Read the model definition and answer for the solid it produces. Units are mm, in the model's axes. Face numbers are marked on the shaded views. A direction names the side the tool comes from. Coordinates: 2 decimals unless noted, no trailing zeros. Write each loop counter-clockwise with the first axis right and the second up, starting at its lowest first coordinate (ties: lowest second). Pieces come first, ordered by that corner, then holes.
(1) The part is cut by section C-C, the plane x = 25.5. Determine the outline of the cut face in (y, z).
(2) The part is cut by section B-B, the plane x = 0. Determine the outline of the cut face in (y, z).
(3) Which of the six approach directions +Z, -Z, +X, -X, +Y, -Y give full straight-line access (tool end or side, diameter ignored) to the marked faces 1, 2, 3 and 4?
(4) The part is cut by section A-A, the plane y = 49. Determine the outline of the cut face in (x, z).
(5) The part is cut by section D-D, the plane x = -25. Determine the outline of the cut face in (y, z).
(6) Determine the mould class of the marked faces 5, 6 and 7 for opening direction Y: pulls with the +Y half, pulls with the -Y half, needs draft (parallel to the pull), parting line crosses it, or undercut.
(7) Straight lines are drawn through the part: line 1 along X through (y, z) = (34.5, 23); line 2 along Y through (x, z) = (-18.5, 29); line 3 along Y through (x, z) = (-8.5, 21). For each, find the intervals that lie inside material, in ascending order.
(8) Given pin 1 (4 mm diameter, centred on x = 2.5, z = 15, fed in from +Y); pin 2 (16.5 mm diameter, centred on x = -5, z = 9, fed in from +Y); pin 3 (5 mm diameter, centred on y = 17, z = 24, fed in from -X); pin 4 (1.5 mm diameter, centred on y = 73.5, z = 11.5, fed in from +X), each flat-ended and moving along its own axis, determine where each tip first touches the part or whether it passes through.
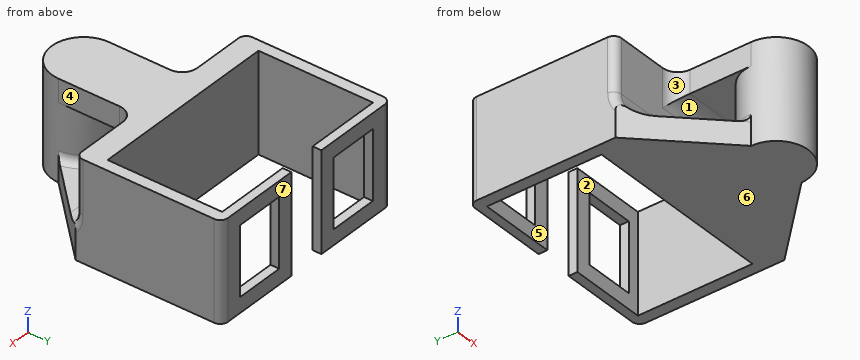
```python
from build123d import *

# Parameters (mm, degrees)
SKETCH1_R             = 10.603707514
BOSS_EXTRUDE1_DEPTH   = 33.02
BOSS_EXTRUDE1_2_DEPTH = 33.02
BOSS_EXTRUDE3_DEPTH   = 7.62
FILLET1_R             = 7.62
FILLET2_START         = 15.24
FILLET2_2_DEPTH       = 18.76
FILLET2_START_2       = -1
FILLET2_3_DEPTH       = 18.231506659
FILLET3_R             = 2.54
SKETCH6_W             = 16.48968
SKETCH6_H             = 22.86
CUT_EXTRUDE1_DEPTH    = 2.905181288
SKETCH7_W             = 21.207415028
SKETCH7_H             = 25.4
BOSS_EXTRUDE4_DEPTH   = 7.62
FILLET4_R             = 5.08


with BuildPart() as part:
    # Sketch1 → Boss-Extrude1 (new body)
    with BuildSketch(Plane.XY):
        Circle(SKETCH1_R)
    extrude(amount=BOSS_EXTRUDE1_DEPTH)



with BuildPart() as body_2:
    # Sketch1 → Boss-Extrude1 2 (new body)
    with BuildSketch(Plane.XY):
        Polygon((-35.51428, 73.999781288), (-35.51428, 25.4), (35.51428, 25.4), (35.51428, 73.999781288), (6.3246, 73.999781288), (6.3246, 71.0946), (31.70428, 71.0946), (31.70428, 33.02), (-31.70428, 33.02), (-31.70428, 71.0946), (-6.3246, 71.0946), (-6.3246, 73.999781288), align=None)
    extrude(amount=BOSS_EXTRUDE1_2_DEPTH)


with BuildPart() as part_1:
    add(part.part)

    add(body_2.part)  # Boss-Extrude3 merges body 2
    # Sketch3 → Boss-Extrude3 (add)
    with BuildSketch(Plane(origin=(0, 0, 0), x_dir=(-1, 0, 0), z_dir=(0, 0, -1))):
        with BuildLine():
            Line((-10.603707514, 0), (-35.51428, 25.4))
            Line((-35.51428, 25.4), (35.51428, 25.4))
            Line((35.51428, 25.4), (10.603707514, 0))
            ThreePointArc((10.603707514, 0), (0, -10.603707514), (-10.603707514, 0))
        make_face()
    extrude(amount=-BOSS_EXTRUDE3_DEPTH)

    # Fillet1
    fillet1_edges = [part_1.edges().sort_by_distance(p)[0] for p in [
        (0, 25.4, 7.62),
    ]]
    fillet(fillet1_edges, radius=FILLET1_R)

    # Fillet2: read off the stored shape, not the designer's step
    # Fillet2 outline → Fillet2 (revolve, cut)
    with BuildSketch(Plane(origin=(0, 17.78, 15.24), x_dir=(0, 1, 0), z_dir=(0, 0, -1))):
        with BuildLine():
            ThreePointArc((10.16, -35.51428), (8.363948776, -34.770331224), (7.62, -32.97428))
            Line((7.62, -32.97428), (7.62, -35.51428))
            Line((7.62, -35.51428), (10.16, -35.51428))
        make_face()
        with BuildLine():
            Line((7.62, 35.51428), (7.62, 32.97428))
            ThreePointArc((7.62, 32.97428), (8.363948776, 34.770331224), (10.16, 35.51428))
            Line((10.16, 35.51428), (7.62, 35.51428))
        make_face()
    revolve(axis=Axis((0, 17.78, 15.24), (1, 0, 0)), mode=Mode.SUBTRACT)

    # Fillet2 2 outline → Fillet2 2 (cut)
    with BuildSketch(Plane.XY.offset(FILLET2_START)):
        with BuildLine():
            Line((-35.51428, 73.999781288), (-35.51428, 71.459781288))
            ThreePointArc((-35.51428, 71.459781288), (-34.770331224, 73.255832512), (-32.97428, 73.999781288))
            Line((-32.97428, 73.999781288), (-35.51428, 73.999781288))
        make_face()
        with BuildLine():
            ThreePointArc((32.97428, 73.999781288), (34.770331224, 73.255832512), (35.51428, 71.459781288))
            Line((35.51428, 71.459781288), (35.51428, 73.999781288))
            Line((35.51428, 73.999781288), (32.97428, 73.999781288))
        make_face()
        with BuildLine():
            ThreePointArc((35.51428, 27.94), (34.770331224, 26.143948776), (32.97428, 25.4))
            Line((32.97428, 25.4), (35.51428, 25.4))
            Line((35.51428, 25.4), (35.51428, 27.94))
        make_face()
        with BuildLine():
            ThreePointArc((-32.97428, 25.4), (-34.770331224, 26.143948776), (-35.51428, 27.94))
            Line((-35.51428, 27.94), (-35.51428, 25.4))
            Line((-35.51428, 25.4), (-32.97428, 25.4))
        make_face()
    extrude(amount=FILLET2_2_DEPTH, mode=Mode.SUBTRACT)

    # Fillet2 3 outline → Fillet2 3 (cut)
    with BuildSketch(Plane.XY.offset(FILLET2_START_2)):
        with BuildLine():
            Line((-35.51428, 73.999781288), (-35.51428, 71.459781288))
            ThreePointArc((-35.51428, 71.459781288), (-34.770331224, 73.255832512), (-32.97428, 73.999781288))
            Line((-32.97428, 73.999781288), (-35.51428, 73.999781288))
        make_face()
        with BuildLine():
            ThreePointArc((32.97428, 73.999781288), (34.770331224, 73.255832512), (35.51428, 71.459781288))
            Line((35.51428, 71.459781288), (35.51428, 73.999781288))
            Line((35.51428, 73.999781288), (32.97428, 73.999781288))
        make_face()
    extrude(amount=FILLET2_3_DEPTH, mode=Mode.SUBTRACT)

    # Fillet3
    # the kernel refuses this fillet: 2.54 mm, written as the material it adds along each edge
    with BuildSketch(Plane(origin=(0, 0, 7.62), x_dir=(-0.8254427651523181, -0.5644858204221742, 0), z_dir=(0.5644858204221742, -0.8254427651523181, 0))) as fillet3_piece_1_section:
        with BuildLine():
            CenterArc((10.603707514 + FILLET3_R, -FILLET3_R), FILLET3_R, 90, 90)
            Line((10.603707514 + FILLET3_R, 0), (10.603707514, 0))
            Line((10.603707514, 0), (10.603707514, -FILLET3_R))
        make_face()
    fillet3_piece_1 = revolve(axis=Axis((0, 0, 7.62), (0, 0, -1)), revolution_arc=248.733186756, mode=Mode.PRIVATE)
    fillet3_piece_1 = split(fillet3_piece_1, bisect_by=Plane(origin=(5.404998183, -5.300850355, 7.62), z_dir=(-0.713951821892461, 0.7001948271848599, 0)), keep=Keep.TOP, mode=Mode.PRIVATE)
    fillet3_piece_1 = split(fillet3_piece_1, bisect_by=Plane(origin=(-5.404998183, -5.300850355, 7.62), z_dir=(0.713951821892461, 0.7001948271848599, 0)), keep=Keep.TOP, mode=Mode.PRIVATE)
    add(fillet3_piece_1)

    # Sketch6 → Cut-Extrude1 (cut)
    with BuildSketch(Plane(origin=(0, 73.999781288, 0), x_dir=(1, 0, 0), z_dir=(0, 1, 0))):
        with Locations((-19.64944, -16.51)):
            Rectangle(SKETCH6_W, SKETCH6_H)
        with Locations((19.64944, -16.51)):
            Rectangle(SKETCH6_W, SKETCH6_H)
    extrude(amount=-CUT_EXTRUDE1_DEPTH, mode=Mode.SUBTRACT)

    # Sketch7 → Boss-Extrude4 (add)
    with BuildSketch(Plane.XY.offset(33.02)):
        with Locations((0, 12.7)):
            Rectangle(SKETCH7_W, SKETCH7_H)
    extrude(amount=-BOSS_EXTRUDE4_DEPTH)

    # Fillet4
    fillet4_edges = [part_1.edges().sort_by_distance(p)[0] for p in [
        (0, 25.4, 25.4),
        (-10.603707514, 25.4, 29.21),
        (10.603707514, 25.4, 29.21),
    ]]
    fillet(fillet4_edges, radius=FILLET4_R)


solid = part_1.part
```
Computed:
1. outline: (15.19, 0) - (33.02, 0) - (33.02, 33.02) - (25.4, 33.02) - (25.4, 15.24) arc R7.62 cw to (17.78, 7.62) - (15.19, 7.62) - close; (71.09, 0) - (74, 0) - (74, 5.08) - (71.09, 5.08) - close; (71.09, 27.94) - (74, 27.94) - (74, 33.02) - (71.09, 33.02) - close
2. outline: (-10.6, 0) - (33.02, 0) - (33.02, 33.02) - (-10.6, 33.02) - close; hole (10.6, 10.16) arc R2.54 ccw to (13.14, 7.62) - (17.78, 7.62) arc R7.62 ccw to (25.4, 15.24) - (25.4, 20.32) arc R5.08 ccw to (20.32, 25.4) - (10.6, 25.4) - close
3. face 1: +X, -X
3. face 2: +Z, -Z
3. face 3: +Z, -X, -Y
3. face 4: +Z, +X, -Y
4. outline: (-35.51, 0) - (-31.7, 0) - (-31.7, 33.02) - (-35.51, 33.02) - close; (31.7, 0) - (35.51, 0) - (35.51, 33.02) - (31.7, 33.02) - close
5. outline: (14.68, 0) - (33.02, 0) - (33.02, 33.02) - (25.4, 33.02) - (25.4, 15.24) arc R7.62 cw to (17.78, 7.62) - (14.68, 7.62) - close; (71.09, 0) - (74, 0) - (74, 5.08) - (71.09, 5.08) - close; (71.09, 27.94) - (74, 27.94) - (74, 33.02) - (71.09, 33.02) - close
6. face 5: undercut
6. face 6: needs draft
6. face 7: pulls with the +Y half
7. line 1: x = -35.51 to -31.7, 31.7 to 35.51
7. line 2: y = 25.4 to 33.02, 71.09 to 74
7. line 3: y = -6.34 to 6.34, 25.35 to 33.02, 71.09 to 74
8. pin 1: stops at y = 33.02
8. pin 2: stops at y = 74
8. pin 3: stops at x = -10.6
8. pin 4: stops at x = 35.16
